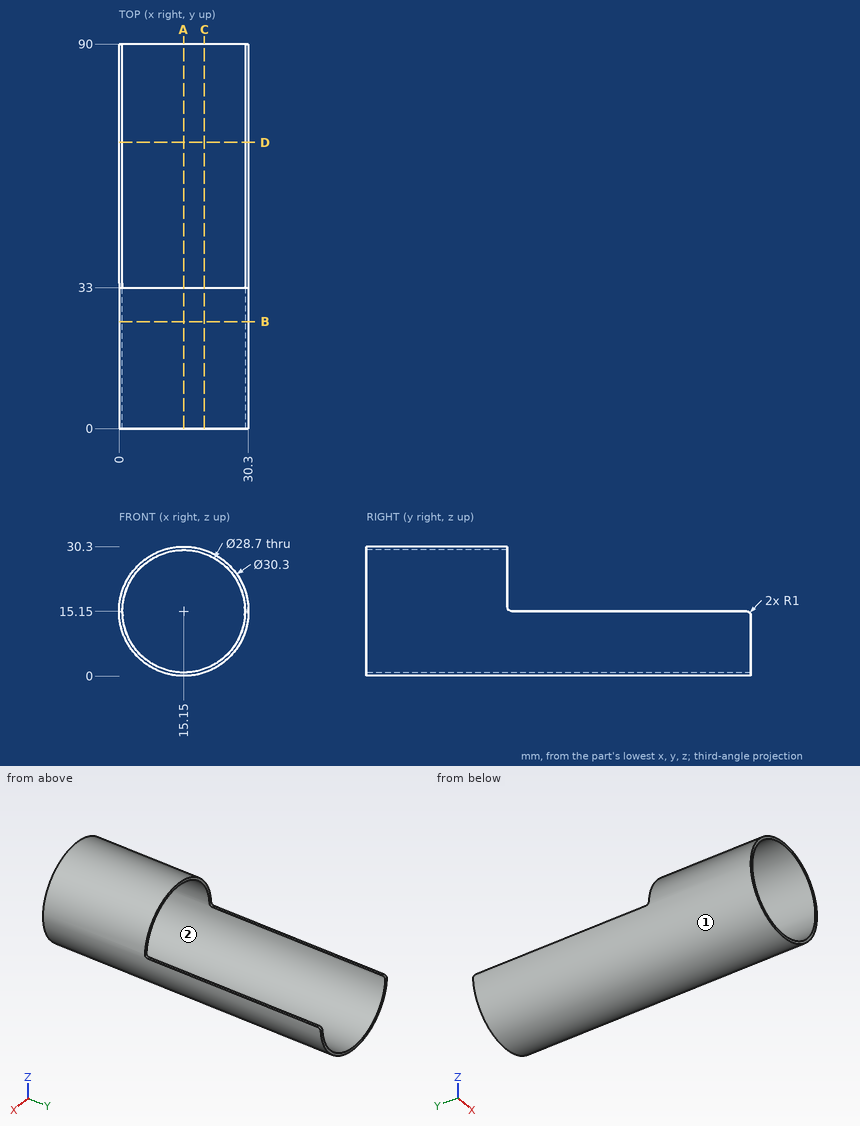
For this review, use the dimensioned drawing (mm, ordinates from the lowest corner) and the shaded views. Give positions to 0.01 mm unless a question says otherwise; leave off trailing zeros. Order: outer loops, then holes, each group sorted by start corner. A loop starts at its lowest first (then second) coordinate and runs counter-clockwise, first axis right, second up. Notation, with made-up numbers: (-33.75, -34) - (-3.75, -34) arc R25 ccw to (-3.75, 1) - close; hole circle Ø5 at (2.25, 1.25). An arc over 180 degrees is marked (long way). Use CSV: the item, a comma, the result in double quotes. Start each with the question number.
Q1. The part is to be moulded in two halves that separate along Z. For the marked faces 1 and 2, say which applies: +Z half, -Z half, draft (parallel to the pull), parting line (faces both ways), or undercut.
Q2. We need section C-C, the plane x = 20. Write out the cut boundary in (y, z), and give its area (3 significant figures).
Q3. Clearance check with flat-ended pins moving along their axes: pin 1 Ø3 at (x, y) = (5.5, 30.5) entering from +Z; pin 2 Ø1 at (x, y) = (19, 48.5) entering from -Z (3 decimals); pin 3 Ø8 at (x, z) = (26.5, 25) entering from +Y; pin 4 Ø4 at (x, z) = (22, 24.5) entering from +Y (3 decimals). State where each tip first meets the part, or that it passes through.
Q4. To check wall thickness, follow line 1 along X through (y, z) = (52, 15); line 2 along Z through (x, y) = (15, 47). State the ranges of each line that lie inside material, in increasing order. Write a range as [from, to].
Q5. We need section B-B, the plane y = 25. Write out the cut boundary in (x, z), and give its area (3 significant figures).
Q6. We need section D-D, the plane y = 67. Write out the cut boundary in (x, z).
Q7. We need section A-A, the plane x = 15.15. Write out the cut boundary in (y, z).
Outcome:
1,face 1,"parting line"
1,face 2,"undercut"
2,outline,"(0, 0.8) - (90, 0.8) - (90, 1.64) - (0, 1.64) - close; (0, 28.66) - (33, 28.66) - (33, 29.5) - (0, 29.5) - close"
2,area,"104 mm^2"
3,pin 1,"stops at z = 27.92"
3,pin 2,"stops at z = 0.375"
3,pin 3,"stops at y = 33"
3,pin 4,"passes through"
4,line 1,"x = [0, 0.8], [29.5, 30.3]"
4,line 2,"z = [0, 0.8]"
5,outline,"circle Ø30.3 at (15.15, 15.15); hole circle Ø28.7 at (15.15, 15.15)"
5,area,"74.1 mm^2"
6,outline,"(0, 15.15) arc R15.15 ccw to (30.3, 15.15) - (29.5, 15.15) arc R14.35 cw to (0.8, 15.15) - close"
7,outline,"(0, 0) - (90, 0) - (90, 0.8) - (0, 0.8) - close; (0, 29.5) - (33, 29.5) - (33, 30.3) - (0, 30.3) - close"
